Solid Edge part; units mm, degrees
sketch "Sketch1" plane through (0, 0, 0) normal (0, 0, 1) x (1, 0, 0)
  circle A0 centre (0, 0) radius 18
extrude "Protrusion1" add sketch "Sketch1" along normal blind 75.6
sketch "Sketch2" plane through (0, 0, 75.6) normal (0, 0, 1) x (1, 0, 0)
  circle A0 centre (0, 0) radius 8
extrude "ExtrudedProtrusion_2" add sketch "Sketch2" along normal blind 6
sketch "Sketch3" plane through (0, 7, 81.6) normal (0, 0, 1) x (1, 0, 0)
  circle A0 centre (0, -7) radius 3
extrude "ExtrudedProtrusion_3" add sketch "Sketch3" along normal blind 15
sketch "Sketch4" plane through (0, 7, 96.6) normal (0, 0, 1) x (1, 0, 0)
  line L0 (-1.6583, -4.5) -> (1.6583, -4.5)
extrude "ExtrudedCutout_1" cut sketch "Sketch4" against normal blind 12 material side at (0, 2.55, 96.6)
hole "Hole_1" at (-7.75, 13.4234, 75.6) direction (0, 0, -1) diameter 3 end through all
pattern_circular "Pattern1" count 6 over 360 about axis through (0, 0, 75.6) along (0, 0, -1) of "Hole_1"
hole "Hole_7" at (26.5, -11.3, 14.25) direction (-1, 0, 0) diameter 0.1 depth 140
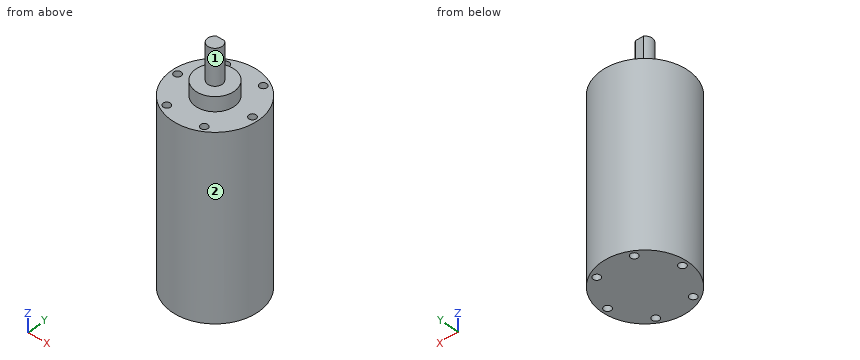
Build history of the part. All positions in model axes, mm. Face numbers are marked on the shaded views. A direction names the side the tool comes from. Round coordinates to 2 decimals unless told otherwise and drop trailing zeros. Loops run counter-clockwise (first coordinate to the right, second up) from the corner with the lowest first, then second, coordinate; pieces in that order, holes last. Notation, with made-up numbers: (-9.75, 68.25) -> (33.25, 68.25) arc R23 cw to (33.25, 107.25) -> close; hole circle Ø2 at (16.5, 73.25). An arc over 180 degrees is marked (long way). Answer in a Markdown table with one row per item.
Item 1: Saw through at C-C (y = 9.5). Write the cut outline in (x, z).
Answers below:
| item | result |
|---|---|
| outline | (-15.29, 0) -> (15.29, 0) -> (15.29, 75.6) -> (-15.29, 75.6) -> close |
Item 2: Saw through at D-D (x = 13). Write the cut outline in (y, z).
Answers below:
| item | result |
|---|---|
| outline | (-12.45, 0) -> (12.45, 0) -> (12.45, 75.6) -> (-12.45, 75.6) -> close; hole circle Ø0.1 at (-11.3, 14.25) |
Item 3: Drill centre lines: L1, parallel to X at y = 13.5, z = 30; L2, parallel to X at y = -1, z = 27.5; L3, parallel to Z at x = -14, y = -4.5. Where is each one in solid material? Low to high. Write a range as [from, to].
Answers below:
| item | result |
|---|---|
| L1 | x = [-11.91, -9.25], [-6.25, 6.25], [9.25, 11.91] |
| L2 | x = [-17.97, -16.62], [-14.38, 14.38], [16.62, 17.97] |
| L3 | z = [0, 75.6] |
Item 4: Which spindle directions (+Z, -Z, +X, -X, +Y, -Y) get a long thin tool onto all of the face, cutting with end or side? Do the marked faces 1 and 2. Say none if no direction does.
Answers below:
| item | result |
|---|---|
| face 1 | +Z |
| face 2 | +Z, -Z |
Item 5: Saw through at A-A (x = 0). Write the cut outline in (y, z), and give its area (3 significant figures).
Answers below:
| item | result |
|---|---|
| outline | (-18, 0) -> (18, 0) -> (18, 75.6) -> (8, 75.6) -> (8, 81.6) -> (3, 81.6) -> (3, 84.6) -> (2.5, 84.6) -> (2.5, 96.6) -> (-3, 96.6) -> (-3, 81.6) -> (-8, 81.6) -> (-8, 75.6) -> (-18, 75.6) -> close; hole circle Ø0.1 at (-11.3, 14.25) |
| area | 2,900 mm² |
Item 6: Saw through at B-B (z = 21). Write the cut outline in (x, y), and give its area (3 significant figures).
Answers below:
| item | result |
|---|---|
| outline | circle Ø36 at (0, 0); hole circle Ø3 at (-15.5, 0); hole circle Ø3 at (-7.75, -13.42); hole circle Ø3 at (-7.75, 13.42); hole circle Ø3 at (7.75, -13.42); hole circle Ø3 at (7.75, 13.42); hole circle Ø3 at (15.5, 0) |
| area | 975 mm² |
Item 7: Pin check, flat tips, straight feed: pin 1 (6 mm diameter, centred on x = -7.5, y = -3, fed in from -Z); pin 2 (2 mm diameter, centred on x = -6, y = -1.5, fed in from +Z); pin 3 (1.5 mm diameter, centred on x = -11, z = 48.5, fed in from -Y); pin 4 (8 mm diameter, centred on y = -13, z = 58, fed in from -X). Stop position of each tip, or through.
Answers below:
| item | result |
|---|---|
| pin 1 | stops at z = 0 |
| pin 2 | stops at z = 81.6 |
| pin 3 | stops at y = -14.8 |
| pin 4 | stops at x = -15.59 |
